Build history of the part. All positions in model axes, mm. Face numbers are marked on the shaded views. A direction names the side the tool comes from. Give positions to 0.01 mm unless a question says otherwise; leave off trailing zeros. Write each loop counter-clockwise with the first axis right and the second up, starting at its lowest first coordinate (ties: lowest second). Pieces come first, ordered by that corner, then holes. Notation, with made-up numbers: (-15, 19) -> (12, 19) arc R13 cw to (12, 30) -> close; hole circle Ø5 at (88.5, -16). An arc over 180 degrees is marked (long way). Write item = value, one per line. Start each with the question number.
Q1. Wall check: line 1 (Y direction, x = 0, z = -5.75); line 2 (Y direction, x = 3.75, z = -5); line 3 (Z direction, x = 0, y = 5). Give the ranges that are in metal, low to high.
Q2. Drop flat-ended pins along their axis: P1, Ø1, axis at x = 5.5, y = 11, coming from the +Z side (3 decimals); P2, Ø3, axis at x = 0, y = 12.5, coming from the -Z side; P3, Ø6, axis at x = 5, y = 6.5, coming from the +Z side; P4, Ø1, axis at x = 4, z = -3, coming from the -Y side. Give the stop position or say it passes through.
Q3. Saw through at A-A, the plane x = 0. List the corners of the cut face in (y, z), then the cut area to 3 significant figures.
Q4. Saw through at C-C, the plane y = 12.5. List the corners of the cut face in (x, z), then the cut area to 3 significant figures.
Q5. Tool access for the marked faces 1, 2 and 3: list every direction of +Z, -Z, +X, -X, +Y, -Y with a clear straight run to the whole face (end or side of a thin tool).
Q6. Mould opens along Y. For the marked faces 4, 5 and 6 say: pulls with the +Y half, pulls with the -Y half, needs draft (parallel to the pull), parting line crosses it, or undercut.
Q7. Saw through at B-B, the plane z = 0. List the corners of the cut face in (x, y), then the cut area to 3 significant figures.
Q8. Saw through at D-D, the plane x = -6. List the corners of the cut face in (y, z), then the cut area to 3 significant figures.
from build123d import *

# Parameters (mm, degrees)
SKETCH1_R           = 8
BOSS_EXTRUDE1_DEPTH = 2
SKETCH2_R           = 5.5
BOSS_EXTRUDE2_DEPTH = 7
SKETCH3_R           = 8
BOSS_EXTRUDE3_DEPTH = 7
SKETCH4_R           = 2.5
CUT_EXTRUDE2_DEPTH  = 17
SKETCH7_R           = 2
CUT_EXTRUDE3_DEPTH  = 9
CIRPATTERN1_COUNT   = 2
CIRPATTERN1_ANGLE   = 90


with BuildPart() as part:
    # Sketch1 → Boss-Extrude1 (new body)
    with BuildSketch(Plane(origin=(0, 0, 0), x_dir=(1, 0, 0), z_dir=(0, 1, 0))):
        Circle(SKETCH1_R)
    extrude(amount=BOSS_EXTRUDE1_DEPTH)

    # Sketch2 → Boss-Extrude2 (add)
    with BuildSketch(Plane(origin=(0, 2, 0), x_dir=(1, 0, 0), z_dir=(0, 1, 0))):
        Circle(SKETCH2_R)
    extrude(amount=BOSS_EXTRUDE2_DEPTH)

    # Sketch3 → Boss-Extrude3 (add)
    with BuildSketch(Plane(origin=(0, 9, 0), x_dir=(1, 0, 0), z_dir=(0, 1, 0))):
        Circle(SKETCH3_R)
    extrude(amount=BOSS_EXTRUDE3_DEPTH)

    # Sketch4 → Cut-Extrude2 (cut, through all)
    with BuildSketch(Plane(origin=(0, 16, 0), x_dir=(1, 0, 0), z_dir=(0, 1, 0))):
        Circle(SKETCH4_R)
    extrude(amount=-CUT_EXTRUDE2_DEPTH, mode=Mode.SUBTRACT)

    # Sketch7 → Cut-Extrude3 (cut, through all)
    with BuildSketch(Plane.XY):
        with Locations((0, 12.5)):
            Circle(SKETCH7_R)
    cut_extrude3 = extrude(amount=-CUT_EXTRUDE3_DEPTH, mode=Mode.SUBTRACT)

    # CirPattern1: Cut-Extrude3 ×2 about axis
    cirpattern1_axis = Axis((0, 16, 0), (0, -1, 0))
    for i in range(1, CIRPATTERN1_COUNT):
        add(cut_extrude3.rotate(cirpattern1_axis, i * CIRPATTERN1_ANGLE / (CIRPATTERN1_COUNT - 1)), mode=Mode.SUBTRACT)


solid = part.part
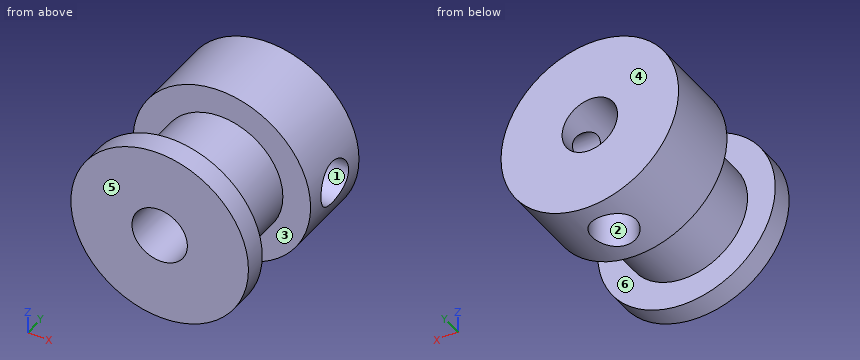
Report:
q1.line_1 = 0 to 2, 9 to 10.5, 14.5 to 16
q1.line_2 = 0 to 2, 9 to 16
q1.line_3 = -5.5 to -2.5, 2.5 to 5.5
q2.P1 = 6.245
q2.P2 = 2
q2.P3 = 7.27
q2.P4 = 0
q3.outline = (0, -8) -> (2, -8) -> (2, -5.5) -> (9, -5.5) -> (9, -8) -> (10.5, -8) -> (10.5, -2.5) -> (0, -2.5) -> close; (0, 2.5) -> (16, 2.5) -> (16, 8) -> (9, 8) -> (9, 5.5) -> (2, 5.5) -> (2, 8) -> (0, 8) -> close; (14.5, -8) -> (16, -8) -> (16, -2.5) -> (14.5, -2.5) -> close
q3.area = 119 mm2
q4.outline = (-2, -7.75) -> (-2, -1.5) arc R2.5 cw to (1.5, 2) -> (7.75, 2) arc R8 ccw (long way) to start; (2, -7.75) arc R8 ccw to (7.75, -2) -> (2, -2) -> close
q4.area = 136 mm2
q5.face_1 = +X
q5.face_2 = -Z
q5.face_3 = none
q6.face_4 = pulls with the +Y half
q6.face_5 = pulls with the -Y half
q6.face_6 = undercut
q7.outline = (-8, 0) -> (-2.5, 0) -> (-2.5, 16) -> (-8, 16) -> (-8, 9) -> (-5.5, 9) -> (-5.5, 2) -> (-8, 2) -> close; (2.5, 0) -> (8, 0) -> (8, 2) -> (5.5, 2) -> (5.5, 9) -> (8, 9) -> (8, 10.5) -> (2.5, 10.5) -> close; (2.5, 14.5) -> (8, 14.5) -> (8, 16) -> (2.5, 16) -> close
q7.area = 119 mm2
q8.outline = (0, -5.29) -> (2, -5.29) -> (2, 5.29) -> (0, 5.29) -> close; (9, -5.29) -> (16, -5.29) -> (16, 5.29) -> (9, 5.29) -> close
q8.area = 95.2 mm2
